from build123d import *

# Parameters (mm, degrees)
POSICIONAMENTOS_R               = 8.2157
BASE_DEPTH                      = 3
FURO_DE_DI_METRO_2_6_2_6_1_D    = 2.6
BASE_DENTE_DEPTH                = 3
RAIO_DENTE_R                    = 1.342367201
PADR_OCIRCULAR1_COUNT           = 8
RAIO_DENTE_OF_PADR_OCIRCULAR1_R = 1.342367201
RESSALTO_EXTRUS_O1_DEPTH        = 3
FURO_DE_DI_METRO_7_3_7_3_1_D    = 7.3


with BuildPart() as part:
    # Posicionamentos → Base (new body)
    with BuildSketch(Plane.XY):
        Circle(POSICIONAMENTOS_R)
    extrude(amount=BASE_DEPTH)

    # Furo de diâmetro Ø2.6 (2.6)1 (through all)
    with Locations(Plane.XY.offset(3)):
        with Locations((0, -6.5), (-6.5, 0)):
            Hole(FURO_DE_DI_METRO_2_6_2_6_1_D / 2)

    # Dente → Base Dente (add, through all)
    with BuildSketch(Plane.XY):
        with BuildLine():
            Line((2.358922349, 10.642131153), (1.777928991, 8.021015833))
            ThreePointArc((1.777928991, 8.021015833), (0, 8.2157), (-1.777928991, 8.021015833))
            Line((-1.777928991, 8.021015833), (-2.358922349, 10.642131153))
            ThreePointArc((-2.358922349, 10.642131153), (-2.364262787, 11.016570047), (-2.263047735, 11.377109253))
            ThreePointArc((-2.263047735, 11.377109253), (-1.685191659, 13.049606095), (-0.650923694, 14.48538223))
            ThreePointArc((-0.650923694, 14.48538223), (0, 14.5), (0.650923694, 14.48538223))
            ThreePointArc((0.650923694, 14.48538223), (1.685191659, 13.049606095), (2.263047735, 11.377109253))
            ThreePointArc((2.263047735, 11.377109253), (2.364262787, 11.016570047), (2.358922349, 10.642131153))
        make_face()
    base_dente = extrude(amount=BASE_DENTE_DEPTH)

    # Raio Dente
    raio_dente_edges = [part.edges().sort_by_distance(p)[0] for p in [
        (-1.777928991, 8.021015833, 1.5),
        (1.777928991, 8.021015833, 1.5),
    ]]
    fillet(raio_dente_edges, radius=RAIO_DENTE_R)

    # PadrãoCircular1: Base Dente ×8 about axis, 2 skipped
    padr_ocircular1_axis = Axis((0, 0, 0), (0, 0, -1))
    add([base_dente.rotate(padr_ocircular1_axis, i * 360 / PADR_OCIRCULAR1_COUNT) for i in range(1, PADR_OCIRCULAR1_COUNT) if i not in (2, 3)])

    # Raio Dente of PadrãoCircular1
    raio_dente_of_padr_ocircular1_edges = [part.edges().sort_by_distance(p)[0] for p in [
        (4.414529041, 6.928900334, 1.5),
        (6.928900334, 4.414529041, 1.5),
        (1.777928991, -8.021015833, 1.5),
        (-1.777928991, -8.021015833, 1.5),
        (-4.414529041, -6.928900334, 1.5),
        (-6.928900334, -4.414529041, 1.5),
        (-8.021015833, -1.777928991, 1.5),
        (-8.021015833, 1.777928991, 1.5),
        (-6.928900334, 4.414529041, 1.5),
        (-4.414529041, 6.928900334, 1.5),
    ]]
    fillet(raio_dente_of_padr_ocircular1_edges, radius=RAIO_DENTE_OF_PADR_OCIRCULAR1_R)

    # Encaixe → Ressalto-extrusão1 (add, through all)
    with BuildSketch(Plane.XY):
        with BuildLine():
            Line((0, 3), (14.900434401, 3))
            ThreePointArc((14.900434401, 3), (17.900434401, 0), (14.900434401, -3))
            Line((14.900434401, -3), (0, -3))
            Line((0, -3), (0, 3))
        make_face()
        with BuildLine():
            Line((10.900434401, 1), (14.900434401, 1))
            ThreePointArc((14.900434401, 1), (15.900434401, 0), (14.900434401, -1))
            Line((14.900434401, -1), (10.900434401, -1))
            ThreePointArc((10.900434401, -1), (9.900434401, 0), (10.900434401, 1))
        make_face(mode=Mode.SUBTRACT)
    extrude(amount=RESSALTO_EXTRUS_O1_DEPTH)

    # Furo de diâmetro Ø7.3 (7.3)1 (through all)
    with Locations(Plane.XY.offset(3)):
        with Locations((0, 0)):
            Hole(FURO_DE_DI_METRO_7_3_7_3_1_D / 2)


solid = part.part
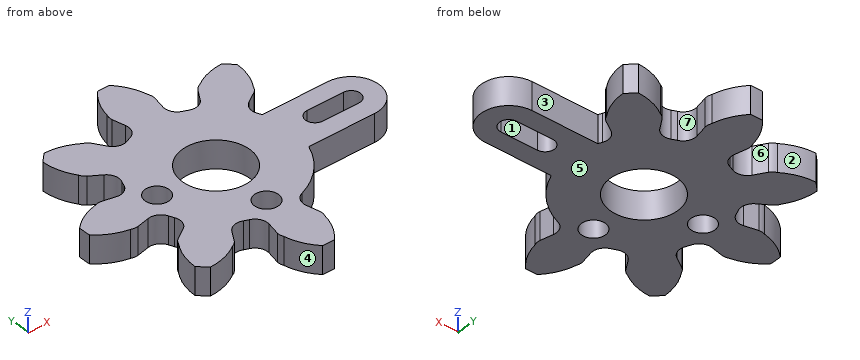
Input: part model. Units: mm. Frame: model coordinates. Face numbers are marked on the shaded views. A direction names the side the tool comes from. Give positions to 0.01 mm unless a question says otherwise; leave off trailing zeros. Loops run counter-clockwise (first coordinate to the right, second up) from the corner with the lowest first, then second, coordinate; pieces in that order, holes last. Notation, with made-up numbers: (67.5, 8) - (75.5, 8) arc R19 cw to (75.5, 21) - close; hole circle Ø7 at (20, 84.5). An arc over 180 degrees is marked (long way). Use CSV: the item, a comma, the result in double quotes. Start each with the question number.
Item 1: Section C-C on z = 1.2. State how many separate pieces and enclosed holes the cut face has, then the cut area to 3 significant figures.
Item 2: Contact query for flat-ended pins moving along their axis: P1, Ø1.5, axis at x = 12.5, z = 1, coming from the -Y side; P2, Ø1, axis at y = 1.5, z = 2, coming from the +X side; P3, Ø2, axis at x = 0, y = -6.5, coming from the -Z side; P4, Ø1, axis at x = 11, z = 0.5, coming from the +Y side. Output: stop coordinate, or through.
Item 3: Section A-A on y = 0. Return loops of the section in (x, z), then the cut area to 3 significant figures.
Item 4: Section D-D on x = 7. Return loops of the section in (y, z), then the cut area to 3 significant figures.
Item 5: Line query: line 1 (Y direction, x = -8.5, z = 2.1); line 2 (Y direction, x = 14, z = 0.9); line 3 (X direction, y = -1.5, z = 0.3). Output: solid intervals per line, ascending.
Item 6: Reachability of the marked faces 1, 2 and 3 from +Z, -Z, +X, -X, +Y, -Y: full face, straight path, thin tool, end or side. Return the list, or none.
Item 7: Section B-B on y = 10.25. Return loops of the section in (x, z).
Item 8: Mould query, pull axis Y, two halves, no side actions, for the marked faces 4, 5, 6 and 7. Classes: pulls with the +Y half, pulls with the -Y half, needs draft (parallel to the pull), parting line crosses it, or undercut.
Ans:
1,separate pieces,"1"
1,enclosed holes,"4"
1,area,"352 mm2"
2,P1,"stops at y = -3"
2,P2,"stops at x = 17.73"
2,P3,"passes through"
2,P4,"stops at y = 10"
3,outline,"(-14.5, 0) - (-7.8, 0) - (-7.8, 3) - (-14.5, 3) - close; (-5.2, 0) - (-3.65, 0) - (-3.65, 3) - (-5.2, 3) - close; (3.65, 0) - (9.9, 0) - (9.9, 3) - (3.65, 3) - close; (15.9, 0) - (17.9, 0) - (17.9, 3) - (15.9, 3) - close"
3,area,"49.5 mm2"
4,outline,"(-4.3, 0) - (9.98, 0) - (9.98, 3) - (-4.3, 3) - close"
4,area,"42.8 mm2"
5,line 1,"y = -10.55 to -5.42, -2.09 to 2.09, 5.42 to 10.55"
5,line 2,"y = -3 to -1, 1 to 3"
5,line 3,"x = -13.38 to -3.33, 3.33 to 17.5"
6,face 1,"+Z, -Z"
6,face 2,"+Z, -Z, +Y"
6,face 3,"+Z, -Z, +X"
7,outline,"(-10.26, 0) - (-7.57, 0) - (-7.57, 3) - (-10.26, 3) - close; (-2.27, 0) - (2.27, 0) - (2.27, 3) - (-2.27, 3) - close; (7.57, 0) - (10.26, 0) - (10.26, 3) - (7.57, 3) - close"
8,face 4,"pulls with the -Y half"
8,face 5,"needs draft"
8,face 6,"pulls with the +Y half"
8,face 7,"undercut"
